CAD build for the part. Positions are in the model's coordinates, mm. Face numbers are marked on the shaded views. A direction names the side the tool comes from. Coordinates: 2 decimals unless noted, no trailing zeros. Loops run counter-clockwise (first coordinate to the right, second up) from the corner with the lowest first, then second, coordinate; pieces in that order, holes last.
1) Two-plate mould, pull along X, no slides. Class the marked faces 5, 6 and 7: +X half, -X half, draft (parallel to the pull), parting line (faces both ways), or undercut.
2) Saw through at A-A, the plane z = 0. Write the cut outline in (x, y), and give its area (3 significant figures).
3) Saw through at B-B, the plane x = 30. Write the cut outline in (y, z), and give its area (3 significant figures).
4) Saw through at D-D, the plane x = -25. Write the cut outline in (y, z).
5) Which spindle directions (+Z, -Z, +X, -X, +Y, -Y) get a long thin tool onto all of the face, cutting with end or side? Do the marked faces 1, 2, 3 and 4. Say none if no direction does.
6) Wall check: line 1 along Z through (x, y) = (3, 12.5); line 2 along X through (y, z) = (7.5, 0); line 3 along X through (y, z) = (4.75, 0). Give the ranges that are in metal, low to high.
7) Pin check, flat tips, straight feed: pin 1 Ø2 at (x, z) = (-19.5, -2) entering from +Y; pin 2 Ø3 at (x, z) = (1, 4.5) entering from -Y; pin 3 Ø3 at (x, z) = (-30, 0) entering from -Y; pin 4 Ø7 at (x, z) = (25.5, 0) entering from +Y. Stop position of each tip, or through.
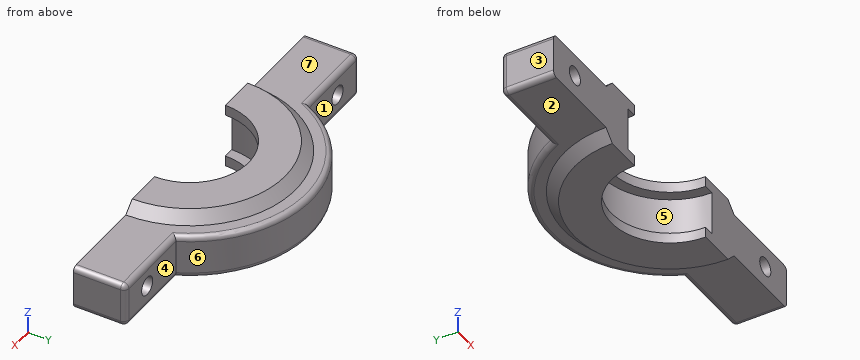
```python
from build123d import *

# Parameters (mm, degrees)
BOSS_EXTRUDE1_DEPTH = 4.2
BOSS_EXTRUDE2_DEPTH = 2
CHAMFER1_SIZE       = 2
SKETCH3_R           = 1.75
CUT_EXTRUDE1_DEPTH  = 40.537861601
FILLET1_R           = 1


with BuildPart() as part:
    # Sketch1 → Boss-Extrude1 (new, symmetric)
    with BuildSketch(Plane.XY):
        with BuildLine():
            Line((36.75, 0), (13.2, 0))
            ThreePointArc((13.2, 0), (0, 13.2), (-13.2, 0))
            Line((-13.2, 0), (-36.75, 0))
            Line((-36.75, 0), (-36.75, 10))
            Line((-36.75, 10), (-20.934182573, 10))
            ThreePointArc((-20.934182573, 10), (0, 23.2), (20.934182573, 10))
            Line((20.934182573, 10), (36.75, 10))
            Line((36.75, 10), (36.75, 0))
        make_face()
    extrude(amount=BOSS_EXTRUDE1_DEPTH, both=True)

    # Sketch2 → Boss-Extrude2 (add)
    with BuildSketch(Plane.XY.offset(4.2)):
        with BuildLine():
            Line((-18.2, 0), (-11.2, 0))
            ThreePointArc((-11.2, 0), (0, 11.2), (11.2, 0))
            Line((11.2, 0), (18.2, 0))
            ThreePointArc((18.2, 0), (0, 18.2), (-18.2, 0))
        make_face()
    boss_extrude2 = extrude(amount=BOSS_EXTRUDE2_DEPTH)

    # Mirror1: Boss-Extrude2 across plane
    add(boss_extrude2.mirror(Plane.XY))

    # Chamfer1
    chamfer1_edges = [part.edges().sort_by_distance(p)[0] for p in [
        (0, 18.2, -4.2),
        (0, 18.2, 4.2),
    ]]
    chamfer(chamfer1_edges, length=CHAMFER1_SIZE - 0.0001)  # a hair under: the kernel refuses the full size

    # Sketch3 → Cut-Extrude1 (cut, through all)
    with BuildSketch(Plane(origin=(0, 10, 0), x_dir=(1, 0, 0), z_dir=(0, 1, 0))):
        with Locations(Location((-30, 0, 0), (0, 0, 270))):
            Circle(SKETCH3_R)
        with Locations(Location((30, 0, 0), (0, 0, 270))):
            Circle(SKETCH3_R)
    extrude(amount=-CUT_EXTRUDE1_DEPTH, mode=Mode.SUBTRACT)

    # Fillet1
    fillet1_edges = [part.edges().sort_by_distance(p)[0] for p in [
        (36.75, 5, -4.2),
        (-36.75, 10, 0),
        (36.75, 10, 0),
        (36.75, 5, 4.2),
        (28.842091287, 10, 4.2),
        (0, 23.2, 4.2),
        (-28.842091287, 10, 4.2),
        (-36.75, 5, 4.2),
        (-36.75, 5, -4.2),
        (-28.842091287, 10, -4.2),
        (0, 23.2, -4.2),
        (28.842091287, 10, -4.2),
    ]]
    fillet(fillet1_edges, radius=FILLET1_R)


solid = part.part
```
Data:
1. face 5: undercut
1. face 6: parting line
1. face 7: draft
2. outline: (-36.75, 0) - (-31.75, 0) - (-31.75, 10) - (-35.75, 10) arc R1 ccw to (-36.75, 9) - close; (-28.25, 0) - (-13.2, 0) arc R13.2 cw to (13.2, 0) - (28.25, 0) - (28.25, 10) - (20.93, 10) arc R23.2 ccw to (-20.93, 10) - (-28.25, 10) - close; (31.75, 0) - (36.75, 0) - (36.75, 9) arc R1 ccw to (35.75, 10) - (31.75, 10) - close
2. area: 787 mm2
3. outline: (0, -4.2) - (9, -4.2) arc R1 ccw to (10, -3.2) - (10, -1.75) - (0, -1.75) - close; (0, 1.75) - (10, 1.75) - (10, 3.2) arc R1 ccw to (9, 4.2) - (0, 4.2) - close
3. area: 48.6 mm2
4. outline: (0, -4.2) - (9, -4.2) arc R1 ccw to (10, -3.2) - (10, 3.2) arc R1 ccw to (9, 4.2) - (0, 4.2) - close
5. face 1: +Z, -Z, -X, +Y
5. face 2: -Z, +Y
5. face 3: +Z, -Z, -X, +Y, -Y
5. face 4: +Z, -Z, +X, +Y
6. line 1: z = -6.2 to -4.2, 4.2 to 6.2
6. line 2: x = -36.75 to -31.75, -28.25 to -10.86, 10.86 to 28.25, 31.75 to 36.75
6. line 3: x = -36.75 to -31.75, -28.25 to -12.32, 12.32 to 28.25, 31.75 to 36.75
7. pin 1: stops at y = 14
7. pin 2: stops at y = 10.92
7. pin 3: passes through
7. pin 4: stops at y = 10
